Source: CAD feature listing. Evaluate the final solid. Frame: model axes, mm. A direction names the side the tool comes from. Round coordinates to 2 decimals unless told otherwise and drop trailing zeros. Loops run counter-clockwise (first coordinate to the right, second up) from the corner with the lowest first, then second, coordinate; pieces in that order, holes last. Notation, with made-up numbers: M -21,64 L 36,64 A37 cw 36,102 Z; hole C 44,19.5 d4. An arc over 180 degrees is marked long. Write each question's results on one line, items separated by ' | '. Start each with the question number.
1. Ray query, line 1 (X direction, y = 108, z = 0); line 2 (Z direction, x = 1, y = 18.5); line 3 (Y direction, x = -11, z = -10). Return the intervals inside material, ascending.
2. Draft query along Z for faces 3 (the flat face through (-5.25, 5, -13.42)), 4 (the flat face through (-12.068, 1.972, -7.098)), 5 (the cylindrical face through (13.137, 125.799, -1.725)), 6 (the flat face through (0, 2, 14)). Return one class per face: released by +Z, released by -Z, zero draft, split by the parting line, or undercut.
3. Section A-A on x = 0. Output: boundary loops of the cut face in (y, z).
4. Section B-B on y = 167. Output: boundary loops of the cut face in (x, z), and give its area (3 significant figures).
5. Contact query for flat-ended pins moving along their axis: pin 1 Ø2 at (x, y) = (12, 127.5) entering from -Z; pin 2 Ø1.5 at (x, y) = (-6, 204) entering from -Z; pin 3 Ø8 at (x, z) = (3.5, 3) entering from -Y; pin 4 Ø6 at (y, z) = (108.5, 13) entering from -X. Output: stop coordinate, or through.
6. Set-up query: faces 1 (the cylindrical face through (5.407, 2.465, 17.169)), 2 (the flat face through (0, 2, -14)). Return all of +Z, -Z, +X, -X, +Y, -Y with unobstructed straight access to the full face (end or side cutting, diameter ignored); none if empty.
from build123d import *

# Parameters (mm, degrees)
SKETCH1_R           = 18
BOSS_EXTRUDE1_DEPTH = 4
SKETCH2_R           = 13.25
SKETCH2_R_2         = 12.25
BOSS_EXTRUDE2_DEPTH = 245
SKETCH3_R           = 18
SKETCH3_R_2         = 12.25
BOSS_EXTRUDE3_DEPTH = 1
CHAMFER1_SIZE       = 1


with BuildPart() as part:
    # Sketch1 → Boss-Extrude1 (new body)
    with BuildSketch(Plane(origin=(0, 0, 0), x_dir=(1, 0, 0), z_dir=(0, 1, 0))):
        with Locations(Location((0, 0, 0), (0, 0, 270))):
            Circle(SKETCH1_R)
        Polygon((8.082903769, -14), (16.165807537, 0), (8.082903769, 14), (-8.082903769, 14), (-16.165807537, 0), (-8.082903769, -14), align=None, mode=Mode.SUBTRACT)
    extrude(amount=BOSS_EXTRUDE1_DEPTH)



with BuildPart() as body_2:
    # Sketch2 → Boss-Extrude2 (new body)
    with BuildSketch(Plane(origin=(0, 4, 0), x_dir=(1, 0, 0), z_dir=(0, 1, 0))):
        with Locations(Location((0, 0, 0), (0, 0, 270))):
            Circle(SKETCH2_R)
        with Locations(Location((0, 0, 0), (0, 0, 270))):
            Circle(SKETCH2_R_2, mode=Mode.SUBTRACT)
    extrude(amount=BOSS_EXTRUDE2_DEPTH)


with BuildPart() as part_1:
    add(part.part)

    add(body_2.part)  # Boss-Extrude3 merges body 2
    # Sketch3 → Boss-Extrude3 (add)
    with BuildSketch(Plane(origin=(0, 4, 0), x_dir=(1, 0, 0), z_dir=(0, 1, 0))):
        with Locations(Location((0, 0, 0), (0, 0, 270))):
            Circle(SKETCH3_R)
        with Locations(Location((0, 0, 0), (0, 0, 270))):
            Circle(SKETCH3_R_2, mode=Mode.SUBTRACT)
    extrude(amount=BOSS_EXTRUDE3_DEPTH)

    # Chamfer1
    chamfer1_edges = [part_1.edges().sort_by_distance(p)[0] for p in [
        (0, 5, -13.25),
    ]]
    chamfer(chamfer1_edges, length=CHAMFER1_SIZE)


solid = part_1.part
Taken from the geometry:
1) line 1: -13.25 to -12.25, 12.25 to 13.25 | line 2: -13.21 to -12.21, 12.21 to 13.21 | line 3: 0 to 5
2) face 3: zero draft | face 4: undercut | face 5: split by the parting line | face 6: undercut
3) outline: M 0,-18 L 5,-18 L 5,-14.25 L 6,-13.25 L 249,-13.25 L 249,-12.25 L 4,-12.25 L 4,-14 L 0,-14 Z; M 0,14 L 4,14 L 4,12.25 L 249,12.25 L 249,13.25 L 6,13.25 L 5,14.25 L 5,18 L 0,18 Z
4) outline: C 0,0 d26.5; hole C 0,0 d24.5 | area: 80.1 mm^2
5) pin 1: z = -7.39 | pin 2: z = -12.17 | pin 3: through | pin 4: x = -8.69
6) face 1: +Y, -Y | face 2: -Y
